Geometry check sheet. Reference: the model listing, model coordinates, mm. Coordinates: 2 decimals unless noted, no trailing zeros. Order: outer loops, then holes, each group sorted by start corner. A loop starts at its lowest first (then second) coordinate and runs counter-clockwise, first axis right, second up. Notation, with made-up numbers: M 63,85.25 L 95,85.25 A24 cw 95,101.25 Z; hole C -21.75,35 d8. An arc over 180 degrees is marked long. One line per item, written item: value. Start each with the question number.
1) Sectioned sample at D-D, the plane y = -60.5. Enter the section's corners in (x, z), then the cut area to 3 significant figures.
2) Sectioned sample at B-B, the plane x = -20. Enter the section's corners in (y, z), then the cut area to 3 significant figures.
3) Thickness scan on L1, parallel to X at y = 51, z = 0.3; L2, parallel to X at y = 21, z = 0.5; L3, parallel to Y at x = -50.7, z = 0.35. Record the ranges inside material, lowest first. Write a range as from..to.
4) Go/stop test with flat-tipped pins: P1, Ø1.8, axis at x = 16.47, y = 49.03, coming from the -Z side; P2, Ø5, axis at x = 50.7, y = -10.25, coming from the -Z side. Record where each tip stops, or that it passes through.
5) Sectioned sample at C-C, the plane z = 0.2. State how many separate pieces and enclosed holes the cut face has, then the cut area to 3 significant figures.
6) Sectioned sample at A-A, the plane y = 0. Enter the section's corners in (x, z).
```python
from build123d import *

# Parameters (mm, degrees)
SKETCH_1_R          = 75
EXTRUDE_1_DEPTH     = 1.2
SKETCH_2_R          = 1.5
CUT_EXTRUDE_1_DEPTH = 107.072805186


with BuildPart() as part:
    # 草图1 → 凸台-拉伸1 (new body)
    with BuildSketch(Plane.XY):
        Circle(SKETCH_1_R)
    extrude(amount=EXTRUDE_1_DEPTH)

    # 草图2 → 切除-拉伸1 (cut, through all)
    with BuildSketch(Plane.XY.offset(1.2)):
        with Locations((-16.473239611, 49.032487972)):
            Circle(SKETCH_2_R)
        with Locations((-6.123239611, 31.105762114)):
            Circle(SKETCH_2_R)
        with Locations((-23.876760389, 20.855762114)):
            Circle(SKETCH_2_R)
        with Locations((-34.226760389, 38.782487972)):
            Circle(SKETCH_2_R)
        with Locations((23.876760389, 20.855762114)):
            Circle(SKETCH_2_R)
        with Locations((6.123239611, 31.105762114)):
            Circle(SKETCH_2_R)
        with Locations((16.473239611, 49.032487972)):
            Circle(SKETCH_2_R)
        with Locations((34.226760389, 38.782487972)):
            Circle(SKETCH_2_R)
        with Locations((30, -10.25)):
            Circle(SKETCH_2_R)
        with Locations((30, 10.25)):
            Circle(SKETCH_2_R)
        with Locations((50.7, 10.25)):
            Circle(SKETCH_2_R)
        with Locations((50.7, -10.25)):
            Circle(SKETCH_2_R)
        with Locations((6.123239611, -31.105762114)):
            Circle(SKETCH_2_R)
        with Locations((23.876760389, -20.855762114)):
            Circle(SKETCH_2_R)
        with Locations((34.226760389, -38.782487972)):
            Circle(SKETCH_2_R)
        with Locations((16.473239611, -49.032487972)):
            Circle(SKETCH_2_R)
        with Locations((-23.876760389, -20.855762114)):
            Circle(SKETCH_2_R)
        with Locations((-6.123239611, -31.105762114)):
            Circle(SKETCH_2_R)
        with Locations((-16.473239611, -49.032487972)):
            Circle(SKETCH_2_R)
        with Locations((-34.226760389, -38.782487972)):
            Circle(SKETCH_2_R)
        with Locations((-30, 10.25)):
            Circle(SKETCH_2_R)
        with Locations((-30, -10.25)):
            Circle(SKETCH_2_R)
        with Locations((-50.7, -10.25)):
            Circle(SKETCH_2_R)
        with Locations((-50.7, 10.25)):
            Circle(SKETCH_2_R)
        with BuildLine():
            ThreePointArc((-18.261036187, 51.880001517), (-24.25, 42.002232084), (-35.798881168, 41.754521996))
            ThreePointArc((-35.798881168, 41.754521996), (-27.5, 47.631397208), (-18.261036187, 51.880001517))
        make_face()
        with BuildLine():
            ThreePointArc((35.798881168, 41.754521996), (24.25, 42.002232084), (18.261036187, 51.880001517))
            ThreePointArc((18.261036187, 51.880001517), (27.5, 47.631397208), (35.798881168, 41.754521996))
        make_face()
        with BuildLine():
            ThreePointArc((54.059917355, -10.125479521), (48.5, 0), (54.059917355, 10.125479521))
            ThreePointArc((54.059917355, 10.125479521), (55, 0), (54.059917355, -10.125479521))
        make_face()
        with BuildLine():
            ThreePointArc((18.261036187, -51.880001517), (24.25, -42.002232084), (35.798881168, -41.754521996))
            ThreePointArc((35.798881168, -41.754521996), (27.5, -47.631397208), (18.261036187, -51.880001517))
        make_face()
        with BuildLine():
            ThreePointArc((-35.798881168, -41.754521996), (-24.25, -42.002232084), (-18.261036187, -51.880001517))
            ThreePointArc((-18.261036187, -51.880001517), (-27.5, -47.631397208), (-35.798881168, -41.754521996))
        make_face()
        with BuildLine():
            ThreePointArc((-54.059917355, 10.125479521), (-48.5, 0), (-54.059917355, -10.125479521))
            ThreePointArc((-54.059917355, -10.125479521), (-55, 0), (-54.059917355, 10.125479521))
        make_face()
    extrude(amount=-CUT_EXTRUDE_1_DEPTH, mode=Mode.SUBTRACT)


solid = part.part
```
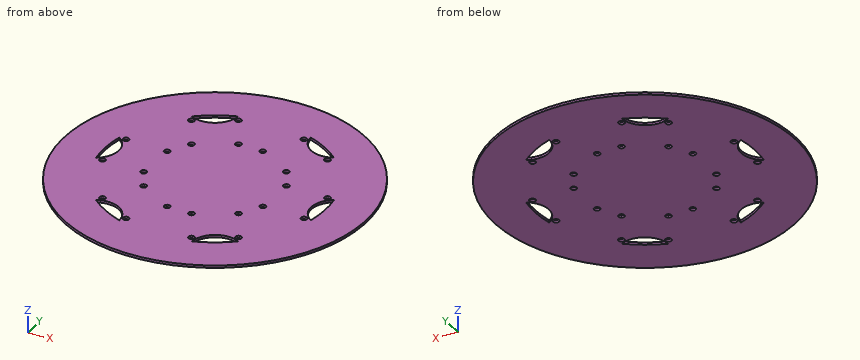
Final values:
1. outline: M -44.33,0 L 44.33,0 L 44.33,1.2 L -44.33,1.2 Z
1. area: 106 mm^2
2. outline: M -72.28,0 L -51.23,0 L -51.23,1.2 L -72.28,1.2 Z; M -46.15,0 L 46.15,0 L 46.15,1.2 L -46.15,1.2 Z; M 51.23,0 L 72.28,0 L 72.28,1.2 L 51.23,1.2 Z
2. area: 161 mm^2
3. L1: x = -54.99..-20.59, -18.33..18.33, 20.59..54.99
3. L2: x = -72..-25.37, -22.38..22.38, 25.37..72
3. L3: y = -55.27..-11.75, -8.75..-6.93, 6.93..8.75, 11.75..55.27
4. P1: passes through
4. P2: stops at z = 0
5. separate pieces: 1
5. enclosed holes: 30
5. area: 16,900 mm^2
6. outline: M -75,0 L -55,0 L -55,1.2 L -75,1.2 Z; M -48.5,0 L 48.5,0 L 48.5,1.2 L -48.5,1.2 Z; M 55,0 L 75,0 L 75,1.2 L 55,1.2 Z
